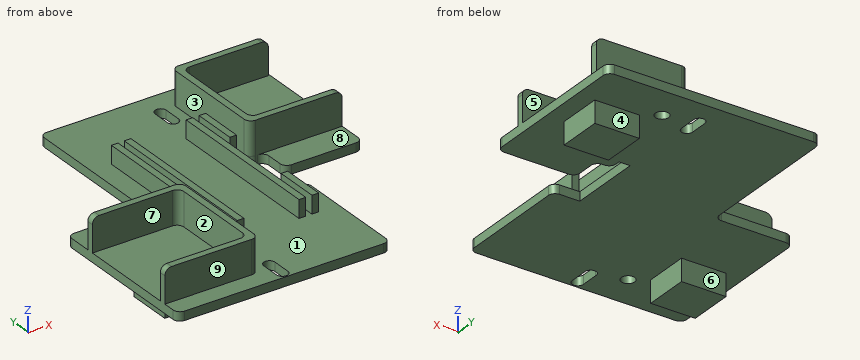
```python
from build123d import *

# Parameters (mm, degrees)
SKETCH3_W             = 1.5
SKETCH3_H             = 36.6
BOSS_EXTRUDE1_DEPTH   = 4
BOSS_EXTRUDE1_2_DEPTH = 4
BOSS_EXTRUDE1_3_DEPTH = 4
BOSS_EXTRUDE1_4_DEPTH = 4
SKETCH4_W             = 65.2
SKETCH4_H             = 70
BOSS_EXTRUDE2_DEPTH   = 2
BOSS_EXTRUDE3_DEPTH   = 7.5
SKETCH6_W             = 17.5
SKETCH6_H             = 29.2
CUT_EXTRUDE1_DEPTH    = 4
SKETCH10_R            = 1.5
CUT_EXTRUDE5_DEPTH    = 20
SKETCH11_W            = 23.629808973
SKETCH11_H            = 13.794178538
SKETCH11_W_2          = 19.491555411
SKETCH11_H_2          = 12.733087881
CUT_EXTRUDE6_DEPTH    = 20
SKETCH13_W            = 4
SKETCH13_H            = 16.6
CUT_EXTRUDE7_DEPTH    = 2
SKETCH15_W            = 6
SKETCH15_H            = 11.6
CUT_EXTRUDE8_DEPTH    = 2
CUT_EXTRUDE9_DEPTH    = 2
FILLET1_R             = 1.5
CUT_EXTRUDE11_DEPTH   = 2
FILLET2_R             = 1.5
SKETCH19_W            = 10
SKETCH19_H            = 10
BOSS_EXTRUDE5_DEPTH   = 4.95


with BuildPart() as part:
    # Sketch3 → Boss-Extrude1 (new body)
    with BuildSketch(Plane.XY):
        with Locations((-6.95, 0)):
            Rectangle(SKETCH3_W, SKETCH3_H)
    extrude(amount=BOSS_EXTRUDE1_DEPTH)



with BuildPart() as body_2:
    # Sketch3 → Boss-Extrude1 2 (new body)
    with BuildSketch(Plane.XY):
        with Locations((-9.85, 0)):
            Rectangle(SKETCH3_W, SKETCH3_H)
    extrude(amount=BOSS_EXTRUDE1_2_DEPTH)


with BuildPart() as body_3:
    # Sketch3 → Boss-Extrude1 3 (new body)
    with BuildSketch(Plane.XY):
        with Locations((6.95, 0)):
            Rectangle(SKETCH3_W, SKETCH3_H)
    extrude(amount=BOSS_EXTRUDE1_3_DEPTH)


with BuildPart() as body_4:
    # Sketch3 → Boss-Extrude1 4 (new body)
    with BuildSketch(Plane.XY):
        with Locations((9.85, 0)):
            Rectangle(SKETCH3_W, SKETCH3_H)
    extrude(amount=BOSS_EXTRUDE1_4_DEPTH)


with BuildPart() as part_1:
    add(part.part)

    add(body_2.part)  # Boss-Extrude2 merges body 2

    add(body_3.part)  # Boss-Extrude2 merges body 3

    add(body_4.part)  # Boss-Extrude2 merges body 4
    # Sketch4 → Boss-Extrude2 (add)
    with BuildSketch(Plane.XY):
        Rectangle(SKETCH4_W, SKETCH4_H)
    extrude(amount=-BOSS_EXTRUDE2_DEPTH)

    # Sketch5 → Boss-Extrude3 (add)
    with BuildSketch(Plane.XY):
        Polygon((11.6, 30.8), (11.6, 5.8), (32.6, 5.8), (32.6, 7.3), (13.1, 7.3), (13.1, 29.3), (32.294650231, 29.3), (32.294650231, 30.8), align=None)
        Polygon((-32.6, -5.8), (-11.6, -5.8), (-11.6, -30.8), (-32.6, -30.8), (-32.6, -29.3), (-13.1, -29.3), (-13.1, -7.3), (-32.6, -7.3), align=None)
    extrude(amount=BOSS_EXTRUDE3_DEPTH)

    # Sketch6 → Cut-Extrude1 (cut)
    with BuildSketch(Plane.XY):
        with Locations((-23.85, 15.4)):
            Rectangle(SKETCH6_W, SKETCH6_H)
        with Locations((23.85, -15.4)):
            Rectangle(SKETCH6_W, SKETCH6_H)
    extrude(amount=-CUT_EXTRUDE1_DEPTH, mode=Mode.SUBTRACT)

    # Sketch10 → Cut-Extrude5 (cut)
    with BuildSketch(Plane(origin=(0, 0, -2), x_dir=(-1, 0, 0), z_dir=(0, 0, -1))):
        with Locations((-15.1, 27.3)):
            Circle(SKETCH10_R)
        with Locations((15.1, -27.3)):
            Circle(SKETCH10_R)
    extrude(amount=-CUT_EXTRUDE5_DEPTH, mode=Mode.SUBTRACT)

    # Sketch11 → Cut-Extrude6 (cut)
    with BuildSketch(Plane.XY):
        with Locations((-26.914904487, 32.734646762)):
            Rectangle(SKETCH11_W, SKETCH11_H)
        with Locations((24.845777706, -31.885774236)):
            Rectangle(SKETCH11_W_2, SKETCH11_H_2)
    extrude(amount=-CUT_EXTRUDE6_DEPTH, mode=Mode.SUBTRACT)

    # Sketch13 → Cut-Extrude7 (cut)
    with BuildSketch(Plane(origin=(10.6, 0, 0), x_dir=(0, 0, -1), z_dir=(1, 0, 0))):
        with Locations((-2, 0)):
            Rectangle(SKETCH13_W, SKETCH13_H)
    extrude(amount=-CUT_EXTRUDE7_DEPTH, mode=Mode.SUBTRACT)

    # Sketch15 → Cut-Extrude8 (cut)
    with BuildSketch(Plane.XY):
        with Locations((12.1, 0)):
            Rectangle(SKETCH15_W, SKETCH15_H)
    extrude(amount=-CUT_EXTRUDE8_DEPTH, mode=Mode.SUBTRACT)

    # Sketch16 → Cut-Extrude9 (cut)
    with BuildSketch(Plane.XY):
        with BuildLine():
            Line((-6.85, -29.3), (-6.85, -33.480622793))
            ThreePointArc((-6.85, -33.480622793), (-8.1, -34.730622793), (-9.35, -33.480622793))
            Line((-9.35, -33.480622793), (-9.33687818, -29.480644316))
            ThreePointArc((-9.33687818, -29.480644316), (-8.190560134, -28.053284771), (-6.85, -29.3))
        make_face()
        with BuildLine():
            Line((6.85, 29.3), (6.85, 25.3))
            ThreePointArc((6.85, 25.3), (8.1, 24.05), (9.35, 25.3))
            Line((9.35, 25.3), (9.35, 29.3))
            ThreePointArc((9.35, 29.3), (8.1, 30.55), (6.85, 29.3))
        make_face()
    extrude(amount=-CUT_EXTRUDE9_DEPTH, mode=Mode.SUBTRACT)

    # Fillet1
    fillet1_edges = [part_1.edges().sort_by_distance(p)[0] for p in [
        (32.6, 6.55, 7.5),
        (32.294650231, 30.05, 7.5),
        (-13.1, -7.3, 3.75),
        (-13.1, -29.3, 3.75),
        (-11.6, -30.8, 3.75),
        (-11.6, -5.8, 3.75),
        (-32.6, -6.55, 7.5),
        (-32.6, -30.05, 7.5),
        (-32.6, 0.8, -1),
        (-15.1, 0.8, -1),
        (32.6, -0.8, -1),
        (15.1, -0.8, -1),
        (-15.1, 35, -1),
        (15.1, -35, -1),
        (15.1, 5.8, -1),
        (15.1, -5.8, -1),
        (32.6, 35, -1),
        (-32.6, -35, -1),
        (11.6, 30.8, 3.75),
        (11.6, 5.8, 3.75),
        (13.1, 7.3, 3.75),
        (13.1, 29.3, 3.75),
    ]]
    fillet(fillet1_edges, radius=FILLET1_R)

    # Sketch18 → Cut-Extrude11 (cut)
    with BuildSketch(Plane.XY):
        Polygon((9.1, 8.3), (11.6, 8.3), (11.6, -5.8), (16.495460275, -5.8), (16.495460275, -8.011234459), (9.1, -8.011234459), align=None)
    extrude(amount=-CUT_EXTRUDE11_DEPTH, mode=Mode.SUBTRACT)

    # Fillet2
    fillet2_edges = [part_1.edges().sort_by_distance(p)[0] for p in [
        (11.6, 5.8, -1),
        (15.1, -8.011234459, -1),
    ]]
    fillet(fillet2_edges, radius=FILLET2_R)

    # Sketch19 → Boss-Extrude5 (add)
    with BuildSketch(Plane(origin=(0, 0, -2), x_dir=(-1, 0, 0), z_dir=(0, 0, -1))):
        with Locations((-23.6, 20)):
            Rectangle(SKETCH19_W, SKETCH19_H)
        with Locations((23.6, -20)):
            Rectangle(SKETCH19_W, SKETCH19_H)
    extrude(amount=BOSS_EXTRUDE5_DEPTH)


solid = part_1.part
```
Can you work these out from the model? Positions are in its coordinate system, mm. Face numbers are marked on the shaded views. A direction names the side the tool comes from. Coordinates: 2 decimals unless noted, no trailing zeros. Loops run counter-clockwise (first coordinate to the right, second up) from the corner with the lowest first, then second, coordinate; pieces in that order, holes last.
Item 1: If we mould it in two halves opening along X, with no side actions, what happens to the marked faces 1, 2, 3 and 4? For each: released by +X, released by -X, zero draft, split by the parting line, or undercut.
Answers below:
face 1: undercut
face 2: released by -X
face 3: undercut
face 4: zero draft
Item 2: Suppose I cut it at A-A (z = -3.75). Please give me the cut outline in (x, y), then the cut area to 3 significant figures.
Answers below:
outline: (-28.6, -25) - (-18.6, -25) - (-18.6, -15) - (-28.6, -15) - close; (18.6, 15) - (28.6, 15) - (28.6, 25) - (18.6, 25) - close
area: 200 mm2
Item 3: Please list where these lines run through material, in increasing order: L1, parallel to X at y = -12.5, z = 3.25; L2, parallel to Y at x = -19, z = 6; L3, parallel to Y at x = 21, z = 1.
Answers below:
L1: x = -13.1 to -11.6, -10.6 to -9.1, -7.7 to -6.2, 6.2 to 7.7, 9.1 to 10.6
L2: y = -30.8 to -29.3, -7.3 to -5.8
L3: y = 5.8 to 7.3, 29.3 to 30.8
Item 4: Suppose I cut it at B-B (x = -22). Please give me the cut outline in (y, z).
Answers below:
outline: (-35, -2) - (-25, -2) - (-25, -6.95) - (-15, -6.95) - (-15, -2) - (0.8, -2) - (0.8, 0) - (-5.8, 0) - (-5.8, 7.5) - (-7.3, 7.5) - (-7.3, 0) - (-29.3, 0) - (-29.3, 7.5) - (-30.8, 7.5) - (-30.8, 0) - (-35, 0) - close
Item 5: Suppose I cut it at C-C (x = -1.5). Please give me the cut outline in (y, z), then the cut area to 3 significant figures.
Answers below:
outline: (-35, -2) - (35, -2) - (35, 0) - (-35, 0) - close
area: 140 mm2
Item 6: I'm going to push flat-ended pins straight in: pin 1 (5 mm diameter, centred on y = 18, z = 1.5, fed in from -X); pin 2 (4 mm diameter, centred on x = -24.5, z = -4.5, fed in from -Y); pin 3 (10 mm diameter, centred on x = -8, y = 12.5, fed in from +Z). Where does each tip first touch, or does it pass through?
Answers below:
pin 1: stops at x = -15.1
pin 2: stops at y = -25
pin 3: stops at z = 4
Item 7: Which directions (+Z, -Z, +X, -X, +Y, -Y) give clear straight access to the entire face, cutting with the end or side of a thin tool? Please do the marked faces 5, 6, 7, 8 and 9.
Answers below:
face 5: +Z, +X
face 6: -Z, +X, -X, +Y
face 7: +Z, -X
face 8: +Z, +X, -Y
face 9: +Z, +X, -X, -Y
